Read the model definition and answer for the solid it produces. Units are mm, in the model's axes. Coordinates: 2 decimals unless noted, no trailing zeros. Loops run counter-clockwise (first coordinate to the right, second up) from the corner with the lowest first, then second, coordinate; pieces in that order, holes last. Notation, with made-up numbers: (81, -7) - (125, -7) arc R28 cw to (125, 16) - close; hole circle Ø5 at (41.5, 47.25). An arc over 180 degrees is marked (long way). Use one line per item in the form item = value. Start each with the question number.
1) Each of these flat-tipped pins is pushed along its axis until it touches: P1, Ø2.5, axis at x = -8.833, z = 57.162, coming from the -Y side; P2, Ø3.5, axis at x = 32.9, z = 46.85, coming from the -Y side; P3, Ø1, axis at x = -28.5, y = 1, coming from the +Z side. Where does it stop, or does it pass through?
2) A cutting plane is placed at B-B (x = 55.5). Give the vertices of the cut face in (y, z).
3) The mould has two halves that part along Z. Classify faces 1 (the face through (86.293, 1.479, 83.591)), 2 (the face through (86.091, 1.479, -83.793)), 3 (the face through (-74.484, 1.406, 12.385)), 4 (the face through (21, 0, -18)): released by +Z, released by -Z, zero draft, split by the parting line, or undercut.
4) A cutting plane is placed at A-A (z = -25.5). Give the vertices of the cut face in (x, y).
5) Consider line 1 (Z direction, x = 0, y = 0.35); line 2 (Z direction, x = 74, y = 2.75); line 3 (Z direction, x = 65, y = 0.35). Determine where each line is inside the solid, lowest interval first.
Autodesk Inventor part; units mm, degrees
ref_plane "YZ Plane" through (0, 0, 0) normal (1, 0, 0) x (0, 1, 0)
ref_plane "XZ Plane" through (0, 0, 0) normal (0, 1, 0) x (-1, 0, 0)
ref_plane "XY Plane" through (0, 0, 0) normal (0, 0, 1) x (1, 0, 0)
sketch "Эскиз1" plane through (0, 0, 0) normal (0, 1, 0) x (-1, 0, 0)
  line L0 (-77, -87.5) -> (77, -87.5)
  line L1 (90, -74.5) -> (90, 74.5)
  line L2 (77, 87.5) -> (-77, 87.5)
  line L3 (-90, 74.5) -> (-90, -74.5)
  line L4 (90, 0) -> (-90, 0) construction
  line L5 (0, -87.5) -> (0, 87.5) construction
  arc A0 (90, 74.5) -> (77, 87.5) centre (77, 74.5) ccw
  arc A1 (77, -87.5) -> (90, -74.5) centre (77, -74.5) ccw
  arc A2 (-90, -74.5) -> (-77, -87.5) centre (-77, -74.5) ccw
  arc A3 (-77, 87.5) -> (-90, 74.5) centre (-77, 74.5) ccw
  line L6 (75, 83.5) -> (-75, 83.5)
  line L7 (-75, 83.5) -> (-75, 65.5)
  line L8 (-75, 65.5) -> (75, 65.5)
  line L9 (75, 65.5) -> (75, 83.5)
  line L10 (0, 87.5) -> (0, -87.5) construction
  line L11 (75, -83.5) -> (-75, -83.5)
  line L12 (-75, -83.5) -> (-75, -65.5)
  line L13 (-75, -65.5) -> (75, -65.5)
  line L14 (75, -65.5) -> (75, -83.5)
  line L15 (90, 49.8397) -> (90, 20.3597)
  line L16 (0, 65.5) -> (42, 65.5)
  line L17 (90, -32.9125) -> (90, 38.6688)
  line L18 (68, 60) -> (-12, 60)
  line L19 (-12, 60) -> (-12, -60)
  line L20 (-12, -60) -> (68, -60)
  line L21 (68, -60) -> (68, 60)
  line L22 (60, 60) -> (57.2, 60)
  line L23 (60, 57.2) -> (60, 60)
  circle A4 centre (65.2, 57.2) radius 1.5
  line L24 (20, 60) -> (20, -60) construction
  circle A5 centre (65.2, -57.2) radius 1.5
  circle A6 centre (-9.2, 57.2) radius 1.5
  circle A7 centre (-9.2, -57.2) radius 1.5
  line L25 (-20, 0) -> (-25, 0) construction
  line L26 (-25, 0) -> (-81, 0) construction
  line L27 (-13, 42.5) -> (-69, 42.5)
  line L28 (-69, 42.5) -> (-69, -42.5)
  line L29 (-69, -42.5) -> (-13, -42.5)
  line L30 (-13, -42.5) -> (-13, 42.5)
  line L31 (-25, 42.5) -> (-28.7, 42.5)
  line L32 (-25, 38.8) -> (-25, 42.5)
  circle A8 centre (-16.7, 38.8) radius 1.5
  line L33 (-53, 42.5) -> (-53, -42.5) construction
  line L34 (-25, 0) -> (-81, 0) construction
  line L35 (-16.7, 38.8) -> (-16.7, -19.2) construction
  circle A9 centre (-16.7, -19.2) radius 1.5
  circle A10 centre (-65.3, 38.8) radius 1.5
  circle A11 centre (-65.3, -19.2) radius 1.5
  line L36 (90, 60.5) -> (90, 65.5)
  circle A12 centre (65, 60.3847) radius 1.5
  circle A13 centre (65, 52.5) radius 1.5
  line L37 (32.5, 60.3847) -> (32.5, -60) construction
  circle A14 centre (0, 60.3847) radius 1.5
  circle A15 centre (0, 52.5) radius 1.5
  circle A16 centre (-65, 60.3847) radius 1.5
  circle A17 centre (-65, 52.5) radius 1.5
  circle A18 centre (65, -60.3847) radius 1.5
  circle A19 centre (65, -52.5) radius 1.5
  circle A20 centre (0, -60.3847) radius 1.5
  circle A21 centre (0, -52.5) radius 1.5
  circle A22 centre (-65, -60.3847) radius 1.5
  circle A23 centre (-65, -52.5) radius 1.5
  circle A24 centre (86, 0) radius 1.5
  line L38 (86, 0) -> (104.385, 0) construction
  circle A25 centre (72.9998, -13.0002) radius 1.5
  circle A26 centre (72.9998, 12.9998) radius 1.5
  line L39 (90, -19.2) -> (75, -19.2)
  line L40 (75, -19.2) -> (75, 22.1472)
  line L41 (75, 22.1472) -> (90, 22.1472)
  line L42 (90, 22.1472) -> (90, -19.2)
  line L43 (-90, 8.1057) -> (-90, 0)
  line L44 (0, 0) -> (-12, 0)
  line L45 (-12, 5.1924) -> (-12, 5.1924)
  line L46 (75, 78.692) -> (75, 65.5)
  circle A27 centre (81.192, 78.692) radius 1.5
  circle A28 centre (81.192, -78.692) radius 1.5
  circle A29 centre (81.192, 68.692) radius 1.5
  circle A30 centre (81.192, -68.692) radius 1.5
  line L47 (66.2, 9.8) -> (66.2, -10.5)
  line L48 (66.2, -10.5) -> (60.2, -10.5)
  line L49 (60.2, -10.5) -> (60.2, 9.8)
  line L50 (60.2, 9.8) -> (66.2, 9.8)
  circle A31 centre (-81.192, -78.692) radius 1.5
  circle A32 centre (-81.192, 78.692) radius 1.5
  line L51 (0, 0) -> (-71.5, 0) construction
  line L52 (-71.5, 0) -> (-71.5, 45.306) construction
  line L53 (-71.5, 45.306) -> (0, 45.306) construction
  line L54 (0, 45.306) -> (0, 0) construction
  line L55 (-71.5, 45.306) -> (-88, 45.306)
  line L56 (-88, 45.306) -> (-88, 62.3062)
  line L57 (-88, 62.3062) -> (-71.5, 62.3062)
  line L58 (-71.5, 62.3062) -> (-71.5, 45.306)
  line L59 (-71.5, -45.306) -> (-88, -45.306)
  line L60 (-88, -45.306) -> (-88, -62.3062)
  line L61 (-88, -62.3062) -> (-71.5, -62.3062)
  line L62 (-71.5, -62.3062) -> (-71.5, -45.306)
  line L63 (20, -40) -> (-20, -40)
  line L64 (-20, -40) -> (-20, 40)
  line L65 (-20, 40) -> (20, 40)
  line L66 (20, 40) -> (20, -40)
  line L67 (20, 0) -> (-20, 0) construction
  line L68 (0, -40) -> (0, 40) construction
  line L69 (0, 65.5) -> (-4.2, 65.5) construction
  line L70 (-4.2, 65.5) -> (-4.2, 56.5) construction
  line L71 (-4.2, 56.5) -> (0, 56.5) construction
  line L72 (0, 56.5) -> (0, 65.5) construction
  circle A33 centre (-4.2, 56.5) radius 1.5
  line L73 (0, 65.5) -> (-29.4, 65.5) construction
  line L74 (-29.4, 65.5) -> (-29.4, 56.5) construction
  line L75 (-29.4, 56.5) -> (0, 56.5) construction
  line L76 (0, 56.5) -> (0, 65.5) construction
  circle A34 centre (-29.4, 56.5) radius 1.5
  circle A35 centre (-4.2, -56.5) radius 1.5
  circle A36 centre (29.4, -56.5) radius 1.5
  line L77 (0, 60.3847) -> (8.833, 60.3847)
  line L78 (8.833, 60.3847) -> (8.833, 57.162)
  line L79 (8.833, 57.162) -> (0, 57.162)
  line L80 (0, 57.162) -> (0, 60.3847)
  circle A37 centre (8.833, 57.162) radius 1.5
  circle A38 centre (-8.833, 57.162) radius 1.5
  circle A39 centre (8.833, -57.162) radius 1.5
  circle A40 centre (-8.833, -57.162) radius 1.5
  line L81 (-20, 0) -> (-20, -8)
  line L82 (-20, -8) -> (-36, -8)
  line L83 (-36, -8) -> (-36, 8)
  line L84 (-36, 8) -> (-20, 8)
  line L85 (-20, 8) -> (-20, -8)
  line L86 (20, -8) -> (36, -8)
  line L87 (36, -8) -> (36, 8)
  line L88 (36, 8) -> (20, 8)
  line L89 (20, 8) -> (20, -8)
  line L90 (0, 0) -> (16.43, 0) construction
  line L91 (16.43, 0) -> (16.43, 43.8) construction
  line L92 (16.43, 43.8) -> (0, 43.8) construction
  line L93 (0, 43.8) -> (0, 0) construction
  circle A41 centre (16.43, 43.8) radius 1.5
  circle A42 centre (-16.43, 43.8) radius 1.5
  circle A43 centre (16.43, -43.8) radius 1.5
  circle A44 centre (-16.43, -43.8) radius 1.5
  line L94 (0, 0) -> (-32.9, 0) construction
  line L95 (-32.9, 0) -> (-32.9, 46.85) construction
  line L96 (-32.9, 46.85) -> (0, 46.85) construction
  line L97 (0, 46.85) -> (0, 0) construction
  circle A45 centre (-32.9, 46.85) radius 1.5
  line L98 (0, -83.5) -> (3, -83.5)
  line L99 (3, -83.5) -> (-3, -83.5)
  line L100 (-3, -83.5) -> (-3, -65.5)
  line L101 (-3, -65.5) -> (3, -65.5)
  line L102 (3, -65.5) -> (3, -83.5)
  line L103 (-3, 83.5) -> (-3, 65.5)
  line L104 (3, 65.5) -> (3, 83.5)
  line L105 (75, 83.5) -> (75, 87.5)
  line L106 (-75, 83.5) -> (-75, 87.5)
  line L107 (75, -83.5) -> (75, -87.5)
  line L108 (-75, -83.5) -> (-75, -87.5)
  point P0 (90, 87.5)
  point P1 (90, -87.5)
  point P2 (-90, 87.5)
  point P3 (-77, -74.5)
  point P4 (60, 0)
  point P5 (75, 0)
  point P6 (60, 0)
  point P7 (-60, 0)
  point P8 (-4, 0)
  point P9 (-5, 0)
  point P10 (-15, 0)
  point P11 (-70, 0)
  point P12 (-14, 0)
  point P13 (-28.7, -19.2)
  point P14 (-17.7, -19.2)
  point P15 (-13, 0)
  point P16 (-14, 0)
  point P17 (-17.6, 40)
  point P18 (-15.8, 40)
  dimension "d0" = 180
  dimension "d1" = 175
  dimension "d2" = 13
  dimension "d7" = 150
  dimension "d8" = 18
  dimension "d13" = 80
  dimension "d14" = 120
  dimension "d21" = 56
  dimension "d22" = 85
  dimension "d25" = 3
  dimension "d26" = 58
  dimension "d27" = 3
  dimension "d30" = 3
  dimension "d32" = 3
  dimension "d33" = 32.5
  dimension "d54" = 3
  dimension "d58" = 3
  dimension "d59" = 3
  dimension "d60" = 15
  dimension "d62" = 12
  dimension "d68" = 3
  dimension "d70" = 3
  dimension "d72" = 20.3
  dimension "d73" = 6
  dimension "d76" = 3
  dimension "d77" = 71.5
  dimension "d78" = 45.306
  dimension "d79" = 40
  dimension "d80" = 80
  dimension "d81" = 4.2
  dimension "d82" = 9
  dimension "d83" = 3
  dimension "d84" = 29.4
  dimension "d85" = 9
  dimension "d86" = 3
  dimension "d87" = 3
  dimension "d88" = 8
  dimension "d89" = 16
  dimension "d90" = 16
  dimension "d91" = 16.43
  dimension "d92" = 43.8
  dimension "d93" = 3
  dimension "d94" = 3
  dimension "d104" = 3
  dimension "d105" = 6
sketch "Эскиз2" plane through (0, 0, 0) normal (0, 1, 0) x (-1, 0, 0)
  line L0 (77, 87.5) -> (-77, 87.5)
  line L1 (-90, 74.5) -> (-90, -74.5)
  line L2 (-77, -87.5) -> (77, -87.5)
  line L3 (90, -74.5) -> (90, 74.5)
  line L4 (90, 0) -> (-90, 0) construction
  line L5 (0, 87.5) -> (0, -87.5) construction
  arc A0 (90, 74.5) -> (77, 87.5) centre (77, 74.5) ccw
  arc A1 (-77, 87.5) -> (-90, 74.5) centre (-77, 74.5) ccw
  arc A2 (-90, -74.5) -> (-77, -87.5) centre (-77, -74.5) ccw
  arc A3 (77, -87.5) -> (90, -74.5) centre (77, -74.5) ccw
  line L6 (150, -150) -> (-150, -150)
  line L7 (-150, -150) -> (-150, 150)
  line L8 (-150, 150) -> (150, 150)
  line L9 (150, 150) -> (150, -150)
  line L10 (150, 0) -> (-150, 0) construction
  line L11 (0, -150) -> (0, 150) construction
  circle A4 centre (0, 0) radius 150
  line L12 (75, -74.5) -> (75, -83.5)
  line L13 (75, -83.5) -> (-75, -83.5)
  line L14 (-75, -83.5) -> (-75, -65.5)
  line L15 (-75, -65.5) -> (75, -65.5)
  line L16 (75, -65.5) -> (75, -83.5)
  line L17 (75, 74.5) -> (75, 83.5)
  line L18 (75, 83.5) -> (-75, 83.5)
  line L19 (-75, 83.5) -> (-75, 65.5)
  line L20 (-75, 65.5) -> (75, 65.5)
  line L21 (75, 65.5) -> (75, 83.5)
  line L22 (0, -65.5) -> (42, -65.5)
  line L23 (42, -65.5) -> (77, -65.5)
  line L24 (77, -65.5) -> (77, -82.3082)
  line L25 (77, -82.3082) -> (42, -82.3082)
  line L26 (77, -65.5) -> (7, -65.5)
  line L27 (7, -65.5) -> (7, -82.3082)
  line L28 (7, -82.3082) -> (77, -82.3082)
  line L29 (77, -82.3082) -> (77, -65.5)
  line L30 (-42, -65.5) -> (-77, -65.5)
  line L31 (-77, -65.5) -> (-77, -82.3082)
  line L32 (-7, -65.5) -> (-7, -82.3082)
  line L33 (-7, -82.3082) -> (-77, -82.3082)
  line L34 (42, -65.5) -> (29.5, -65.5)
  line L35 (29.5, -10.5) -> (54.5, -10.5)
  line L36 (54.5, -10.5) -> (54.5, -65.5)
  line L37 (54.5, -65.5) -> (29.5, -65.5)
  line L38 (29.5, -65.5) -> (29.5, -10.5)
  line L39 (29.5, 10.5) -> (54.5, 10.5)
  line L40 (54.5, 10.5) -> (54.5, 65.5)
  line L41 (29.5, 65.5) -> (29.5, 10.5)
  line L42 (-29.5, -10.5) -> (-54.5, -10.5)
  line L43 (-54.5, -10.5) -> (-54.5, -65.5)
  line L44 (-29.5, -65.5) -> (-29.5, -10.5)
  line L45 (-29.5, 65.5) -> (-29.5, 10.5)
  line L46 (-29.5, 10.5) -> (-54.5, 10.5)
  line L47 (-54.5, 10.5) -> (-54.5, 65.5)
  point P0 (0, 0)
  point P1 (-90, -87.5)
  point P2 (-90, 87.5)
  point P3 (90, -87.5)
  point P4 (-80.411, -84.4848)
  point P5 (77, 74.5)
  point P6 (-7, -73.9041)
  point P7 (7, -73.9041)
  dimension "d34" = 180
  dimension "d35" = 175
  dimension "d36" = 13
  dimension "d37" = 300
  dimension "d38" = 300
  dimension "d41" = 150
  dimension "d42" = 18
  dimension "d44" = 35
  dimension "d45" = 70
  dimension "d46" = 14
  dimension "d47" = 84
  dimension "d50" = 25
extrude "Выдавливание1" add sketch "Эскиз1" along normal blind 3 contours A2 L3 A3 L2 L106 L7 L8 L9 L105 A0 L1 L41 L40 L39 A1 L0 L107 L14 L13 L12 L108 | L39 L40 L41 L1 | L18 A12 L21 L20 A18 A20 L19 L63 L66 L86 L87 L88 L65 A14 L80 L79 A37 L78 | L78 A37 L79 L80 A14 L18 | L18 A14 L77 L78 | L65 A8 L64 L84 L83 L82 L63 L30 L29 A44 L28 L27 A42 | L65 A8 | A4 | A5 | A38 A6 | A40 A7 | A10 | A11 picked at (-16.908, 40.0547) picked at (-10.5675, 57.2211) picked at (-10.5675, -57.2211)
chamfer "Фаска3" distance 1.7 angle 45 22 edges at (-63.5, 3, 52.5) (-63.5, 3, 60.3847) (1.5, 3, 52.5) (1.5, 3, 60.3847) (66.5, 3, 52.5) (66.5, 3, 60.3847) (66.5, 3, -60.3847) (66.5, 3, -52.5) (1.5, 3, -60.3847) (1.5, 3, -52.5) (-63.5, 3, -52.5) (-63.5, 3, -60.3847) (-71.4998, 3, 12.9998) (-84.5, 3, 0) (-71.4998, 3, -13.0002) (34.4, 0, 46.85) (-79.692, 0, 78.692) (-79.692, 0, 68.692) (82.692, 0, 78.692) (82.692, 0, -78.692) (-79.692, 0, -78.692) (-79.692, 0, -68.692)
properties part number "base"
Found:
q1.P1 = through
q1.P2 = 1.45
q1.P3 = 65.5
q2.outline = (0, -65.5) - (3, -65.5) - (3, 65.5) - (0, 65.5) - close
q3.face_1 = released by +Z
q3.face_2 = released by -Z
q3.face_3 = undercut
q3.face_4 = zero draft
q4.outline = (-90, 0) - (-20, 0) - (-20, 3) - (-90, 3) - close; (20, 0) - (90, 0) - (90, 3) - (20, 3) - close
q5.line_1 = -65.5 to -61.88, -58.88 to -54, -51 to -40, 40 to 51, 54 to 58.88, 61.88 to 65.5
q5.line_2 = -65.5 to -62.31, -45.31 to 45.31, 62.31 to 65.5
q5.line_3 = -65.5 to -61.88, -58.88 to -54, -51 to 51, 54 to 58.88, 61.88 to 65.5
